```python
from build123d import *

# Parameters (mm, degrees)
PAD_DEPTH       = 112
SKETCH001_W     = 56
SKETCH001_H     = 10
SKETCH001_H_2   = 15
POCKET_DEPTH    = 5.001
POCKET001_DEPTH = 106
SKETCH003_R     = 1.25
POCKET002_DEPTH = 5.001
POCKET003_DEPTH = 5.001
SKETCH005_R     = 1.8
POCKET004_DEPTH = 2
SKETCH006_W     = 60
SKETCH006_H     = 1
PAD001_DEPTH    = 1


with BuildPart() as part:
    # Sketch → Pad (new body)
    with BuildSketch(Plane.XZ):
        with BuildLine():
            ThreePointArc((-35, 5), (-37.5, 2.5), (-35, 0))
            Line((-35, 0), (35, 0))
            ThreePointArc((35, 0), (37.5, 2.5), (35, 5))
            Line((-35, 5), (35, 5))
        make_face()
    extrude(amount=PAD_DEPTH)

    # Sketch001 (on DatumPlane) → Pocket (cut, through all)
    with BuildSketch(Plane(origin=(0, 0, 5), x_dir=(-1, 0, 0), z_dir=(0, 0, 1))):
        with Locations((0, 103)):
            Rectangle(SKETCH001_W, SKETCH001_H)
        with Locations((0, 85.5)):
            Rectangle(SKETCH001_W, SKETCH001_H_2)
        with Locations((0, 68.5)):
            Rectangle(SKETCH001_W, SKETCH001_H_2)
        with Locations((0, 51.5)):
            Rectangle(SKETCH001_W, SKETCH001_H_2)
        with Locations((0, 34.5)):
            Rectangle(SKETCH001_W, SKETCH001_H_2)
        with Locations((0, 17.5)):
            Rectangle(SKETCH001_W, SKETCH001_H_2)
    extrude(amount=-POCKET_DEPTH, mode=Mode.SUBTRACT)

    # Sketch002 (on DatumPlane) → Pocket001 (cut)
    with BuildSketch(Plane.XZ.offset(112)):
        Polygon((-30, 9), (30, 9), (30, 4), (32, 2.6), (32, 2), (30, 2), (30, 1), (-30, 1), (-30, 2), (-32, 2), (-32, 2.6), (-30, 4), align=None)
    extrude(amount=-POCKET001_DEPTH, mode=Mode.SUBTRACT)

    # Sketch003 (on DatumPlane) → Pocket002 (cut, through all)
    with BuildSketch(Plane(origin=(0, 0, 5), x_dir=(-1, 0, 0), z_dir=(0, 0, 1))):
        with Locations((33, 85.5)):
            Circle(SKETCH003_R)
        Polygon((-38, 20), (-33, 17.5), (-38, 15), align=None)
        Polygon((-38, 32), (-33, 34.5), (-38, 37), align=None)
        Polygon((38, 20), (33, 17.5), (38, 15), align=None)
        Polygon((-38, 54), (-38, 49), (-33, 51.5), align=None)
        Polygon((-38, 71), (-38, 66), (-33, 68.5), align=None)
        Polygon((-38, 88), (-38, 83), (-33, 85.5), align=None)
        Polygon((38, 32), (38, 37), (33, 34.5), align=None)
        Polygon((38, 49), (38, 54), (33, 51.5), align=None)
        Polygon((38, 66), (38, 71), (33, 68.5), align=None)
        Polygon((-1, 0), (1, 0), (1, 3), (-7, 3), (-1, 2), align=None)
    extrude(amount=-POCKET002_DEPTH, mode=Mode.SUBTRACT)

    # Sketch004 (on DatumPlane) → Pocket003 (cut, through all)
    with BuildSketch(Plane(origin=(0, 0, 0), x_dir=(1, 0, 0), z_dir=(0, 0, -1))):
        with BuildLine():
            ThreePointArc((-37.5, 4), (-36.328427, 1.171573), (-33.5, 0))
            Line((-37.5, 0), (-33.5, 0))
            Line((-37.5, 4), (-37.5, 0))
        make_face()
        with BuildLine():
            ThreePointArc((33.5, 0), (36.328427, 1.171573), (37.5, 4))
            Line((37.5, 0), (37.5, 4))
            Line((33.5, 0), (37.5, 0))
        make_face()
        with BuildLine():
            ThreePointArc((-33.5, 112), (-36.328427, 110.828427), (-37.5, 108))
            Line((-37.5, 112), (-37.5, 108))
            Line((-33.5, 112), (-37.5, 112))
        make_face()
        with BuildLine():
            ThreePointArc((37.5, 108), (36.328427, 110.828427), (33.5, 112))
            Line((33.5, 112), (37.5, 112))
            Line((37.5, 112), (37.5, 108))
        make_face()
    extrude(amount=-POCKET003_DEPTH, mode=Mode.SUBTRACT)

    # Sketch005 (on DatumPlane) → Pocket004 (cut)
    with BuildSketch(Plane(origin=(0, 0, 5), x_dir=(-1, 0, 0), z_dir=(0, 0, 1))):
        with Locations((33, 85.5)):
            Circle(SKETCH005_R)
    extrude(amount=-POCKET004_DEPTH, mode=Mode.SUBTRACT)

    # Sketch006 (on DatumPlane) → Pad001 (join)
    with BuildSketch(Plane(origin=(0, 0, 1), x_dir=(-1, 0, 0), z_dir=(0, 0, 1))):
        with Locations((0, 111.5)):
            Rectangle(SKETCH006_W, SKETCH006_H)
    extrude(amount=PAD001_DEPTH)


solid = part.part
```
Geometry: final body of the model. Coordinates: model frame, mm. A direction names the side the tool comes from. Give positions to 0.01 mm unless a question says otherwise; leave off trailing zeros. Write each question's results on one line, items separated by ' | '. Start each with the question number.
1) Line query: line 1 (X direction, y = -79, z = 2.6); line 2 (Y direction, x = 29, z = 1.85); line 3 (Y direction, x = -12.5, z = 2.2). Output: solid intervals per line, ascending. Write a range as from..to.
2) Section A-A (x = -5.5). Count the separate pieces of the cut face and the enclosed holes in it, then the cut area to 3 significant figures.
3) First-contact query: pin 1 (0.8 mm diameter, centred on y = -74.5, z = 1.5, fed in from -X); pin 2 (0.5 mm diameter, centred on y = -60.5, z = 4.5, fed in from +X); pin 3 (0.8 mm diameter, centred on y = -31.5, z = 0.5, fed in from -X); pin 4 (5 mm diameter, centred on x = -25, y = -87, fed in from +Z). Flat tips, straight axial feed; report the tip coordinate or a pass-through.
4) Set-up query: faces 1 (the flat face through (-33, -84, 3)), 2 (the cylindrical face through (37.5, -25.9, 2.4)). Return all of +Z, -Z, +X, -X, +Y, -Y with unobstructed straight access to the full face (end or side cutting, diameter ignored); none if empty.
5) Draft query along X for faces 3 (the cylindrical face through (37.5, -8.3, 2.4)), 4 (the cylindrical face through (-37.5, -8.3, 2.6)), 5 (the flat face through (3, -3, 3)). Return one class per face: pulls with the +X half, pulls with the -X half, needs draft (parallel to the pull), parting line crosses it, or undercut.
Calculated:
1) line 1: -37.5..-32, 32..37.5 | line 2: -112..-111, -6..0 | line 3: -6..0
2) separate pieces: 7 | enclosed holes: 0 | area: 52.0 mm2
3) pin 1: x = -37.43 | pin 2: x = 36.79 | pin 3: x = -36.92 | pin 4: through
4) face 1: +Z | face 2: +X, +Y, -Y
5) face 3: pulls with the +X half | face 4: pulls with the -X half | face 5: undercut
